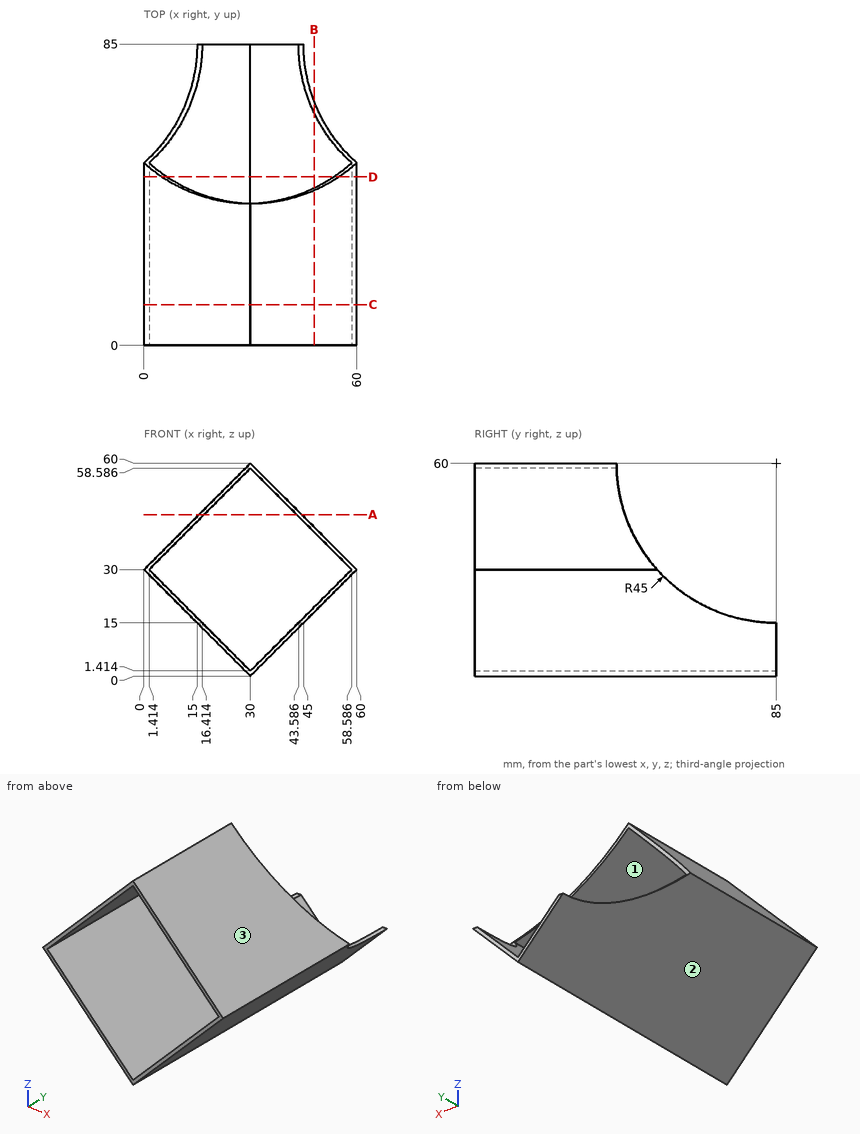
The figure shows three views and two pictorial views of one solid part (mm, origin at its lowest corner). Answer the questions. Coordinates: 2 decimals unless noted, no trailing zeros. Write each loop counter-clockwise with the first axis right and the second up, starting at its lowest first coordinate (ties: lowest second). Pieces come first, ordered by that corner, then holes.
1. Flat-ended cylindrical pins translate along their axes: pin 1 (4 mm diameter, centred on y = 45.5, z = 8.5, fed in from +X); pin 2 (5 mm diameter, centred on x = 16, y = 16.5, fed in from -Z); pin 3 (8 mm diameter, centred on x = 20.5, y = 22, fed in from -Z). Find the tip coordinate at first contact, or state that the pin passes through.
Results list:
pin 1: stops at x = 40.5
pin 2: stops at z = 11.5
pin 3: stops at z = 5.5
2. The part is cut by section D-D, the plane y = 47.5. Write down the section's boundary in (x, z) (1 decimal).
Results list:
outline: (0, 30) - (30, 0) - (60, 30) - (54.9, 35.1) - (53.5, 35.1) - (58.6, 30) - (30, 1.4) - (1.4, 30) - (6.5, 35.1) - (5.1, 35.1) - close
3. For a pull along Z with two mould halves and no side action, classify the marked faces 1, 2 and 3 as +Z half, -Z half, draft (parallel to the pull), parting line (faces both ways), or undercut.
Results list:
face 1: undercut
face 2: -Z half
face 3: +Z half
4. Consider line 1 along X through (y, z) = (69.5, 5) (1 decimal); line 2 along Z through (x, y) = (41, 30) (1 decimal); line 3 along Z through (x, y) = (31.5, 18.5) (1 decimal). Determine where each line is inside the solid, lowest interval first.
Results list:
line 1: x = 25 to 26.4, 33.6 to 35
line 2: z = 11 to 12.4, 47.6 to 49
line 3: z = 1.5 to 2.9, 57.1 to 58.5
5. The part is cut by section B-B, the plane x = 48. Write down the section's boundary in (y, z).
Results list:
outline: (0, 18) - (68.84, 18) arc R45 cw to (65.56, 19.41) - (0, 19.41) - close; (0, 40.59) - (44.4, 40.59) arc R45 cw to (43.76, 42) - (0, 42) - close
6. The part is cut by section A-A, the plane z = 45.5. Write down the section's boundary in (x, y).
Results list:
outline: (15.5, 0) - (16.91, 0) - (16.91, 42.4) - (15.5, 42.4) - close; (43.09, 0) - (44.5, 0) - (44.5, 42.4) - (43.09, 42.4) - close
7. The part is cut by section C-C, the plane y = 11.5. Write down the section's boundary in (x, z).
Results list:
outline: (0, 30) - (30, 0) - (60, 30) - (30, 60) - close; hole (1.41, 30) - (30, 1.41) - (58.59, 30) - (30, 58.59) - close
